from build123d import *

# Parameters (mm, degrees)
SKETCH1_W               = 82.55
SKETCH1_H               = 31.75
BOSS_EXTRUDE1_DEPTH     = 45.72
SHELL1_T                = -1.524
SKETCH3_W               = 25.4
SKETCH3_H               = 5.842
BOSS_EXTRUDE3_DEPTH     = 1.524
FILLET2_R               = 1.27
FILLET3_R               = 1.905
F_2_CLEARANCE_HOLE1_D   = 2.4384
SKETCH6_W               = 44.196
SKETCH6_H               = 28.702
CUT_EXTRUDE1_DEPTH      = 82.026
CUT_EXTRUDE1_DEPTH_BACK = 2.524
FILLET4_R               = 3.556
FILLET5_R               = 5.08
BOSS_EXTRUDE4_DEPTH     = 1.524
FILLET9_R               = 2.54
FILLET10_R              = 2.54


with BuildPart() as part:
    # Sketch1 → Boss-Extrude1 (new body)
    with BuildSketch(Plane.XY):
        Rectangle(SKETCH1_W, SKETCH1_H)
    extrude(amount=BOSS_EXTRUDE1_DEPTH)

    # Shell1
    shell1_openings = [part.faces().sort_by_distance(p)[0] for p in [
        (0, 0, 0),
    ]]
    offset(amount=SHELL1_T, openings=shell1_openings, kind=Kind.INTERSECTION)

    # Sketch3 → Boss-Extrude3 (add)
    with BuildSketch(Plane(origin=(0, 0, 0), x_dir=(-1, 0, 0), z_dir=(0, 0, -1))):
        with Locations((0, 18.796)):
            Rectangle(SKETCH3_W, SKETCH3_H)
        with Locations((0, -18.796)):
            Rectangle(SKETCH3_W, SKETCH3_H)
    extrude(amount=-BOSS_EXTRUDE3_DEPTH)

    # Fillet2
    fillet2_edges = [part.edges().sort_by_distance(p)[0] for p in [
        (12.7, 15.875, 0.762),
        (0, 15.875, 1.524),
        (-12.7, 15.875, 0.762),
        (0, -15.875, 1.524),
        (12.7, -15.875, 0.762),
        (-12.7, -15.875, 0.762),
    ]]
    fillet(fillet2_edges, radius=FILLET2_R)

    # Fillet3
    fillet3_edges = [part.edges().sort_by_distance(p)[0] for p in [
        (12.7, 21.717, 0.762),
        (-12.7, 21.717, 0.762),
        (12.7, -21.717, 0.762),
        (-12.7, -21.717, 0.762),
    ]]
    fillet(fillet3_edges, radius=FILLET3_R)

    # #2 Clearance Hole1 (through all)
    with Locations(Plane.XY.offset(1.524)):
        with Locations((0, 19.431), (0, -19.431)):
            Hole(F_2_CLEARANCE_HOLE1_D / 2)

    # Sketch6 → Cut-Extrude1 (cut, two sides)
    with BuildSketch(Plane(origin=(-39.751, 0, 0), x_dir=(0, 0, -1), z_dir=(1, 0, 0))) as cut_extrude1_sk:
        with Locations((-22.098, 0)):
            Rectangle(SKETCH6_W, SKETCH6_H)
    extrude(amount=CUT_EXTRUDE1_DEPTH, mode=Mode.SUBTRACT)
    extrude(cut_extrude1_sk.sketch, amount=-CUT_EXTRUDE1_DEPTH_BACK, mode=Mode.SUBTRACT)

    # Fillet4
    fillet4_edges = [part.edges().sort_by_distance(p)[0] for p in [
        (0, -14.351, 44.196),
        (0, 14.351, 44.196),
    ]]
    fillet(fillet4_edges, radius=FILLET4_R)

    # Fillet5
    fillet5_edges = [part.edges().sort_by_distance(p)[0] for p in [
        (0, 15.875, 45.72),
        (0, -15.875, 45.72),
    ]]
    fillet(fillet5_edges, radius=FILLET5_R)

    # Sketch7 → Boss-Extrude4 (add)
    with BuildSketch(Plane(origin=(41.275, 0, 0), x_dir=(0, 0, -1), z_dir=(1, 0, 0))):
        with BuildLine():
            Line((-45.72, 10.795), (-45.72, -10.795))
            ThreePointArc((-45.72, -10.795), (-44.232102448, -14.387102448), (-40.64, -15.875))
            Line((-40.64, -15.875), (0, -15.875))
            Line((0, -15.875), (0, -8.89))
            Line((0, -8.89), (-44.196, -8.89))
            Line((-44.196, -8.89), (-44.196, 8.89))
            Line((-44.196, 8.89), (0, 8.89))
            Line((0, 8.89), (0, 15.875))
            Line((0, 15.875), (-40.64, 15.875))
            ThreePointArc((-40.64, 15.875), (-44.232102448, 14.387102448), (-45.72, 10.795))
        make_face()
    boss_extrude4 = extrude(amount=-BOSS_EXTRUDE4_DEPTH)

    # Fillet9
    fillet9_edges = [part.edges().sort_by_distance(p)[0] for p in [
        (40.513, 8.89, 44.196),
        (40.513, -8.89, 44.196),
    ]]
    fillet(fillet9_edges, radius=FILLET9_R)

    # Mirror1: Boss-Extrude4 across plane
    add(boss_extrude4.mirror(Plane(origin=(0, 0, 0), x_dir=(0, 0, 1), z_dir=(1, 0, 0))))

    # Fillet10
    fillet10_edges = [part.edges().sort_by_distance(p)[0] for p in [
        (-40.513, -8.89, 44.196),
        (-40.513, 8.89, 44.196),
    ]]
    fillet(fillet10_edges, radius=FILLET10_R)


solid = part.part
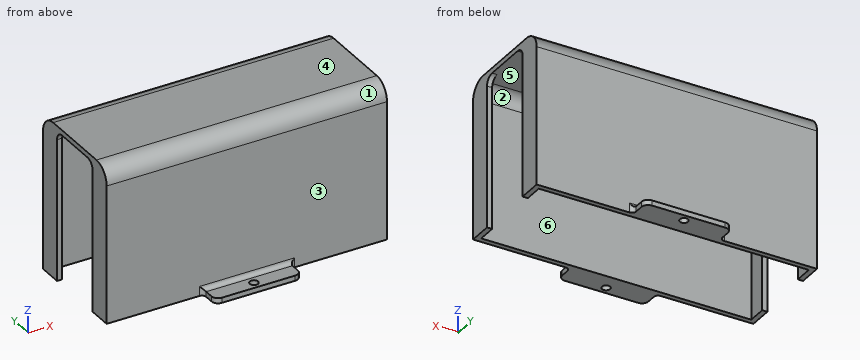
Geometry: final body of the model. Coordinates: model frame, mm. Face numbers are marked on the shaded views. A direction names the side the tool comes from. Coordinates: 2 decimals unless noted, no trailing zeros. Write each loop counter-clockwise with the first axis right and the second up, starting at its lowest first coordinate (ties: lowest second). Pieces come first, ordered by that corner, then holes. Notation, with made-up numbers: (55, 55) - (105, 55) arc R23 ccw to (105, 67) - close; hole circle Ø5 at (51, 52.25). An arc over 180 degrees is marked (long way). Return JSON: item names as keys, results as strings.
Item 1: Pin query (flat end, axial travel): pin 1 Ø3 at (x, y) = (0, -19.431) entering from +Z; pin 2 Ø2 at (y, z) = (7, 38) entering from +X; pin 3 Ø4 at (x, z) = (-24.5, 16.5) entering from -Y (3 decimals); pin 4 Ø0.8 at (y, z) = (19, 0.5) entering from +X. Return the tip coordinate at first contact, or that it passes through.
Completed:
{"pin 1": "stops at z = 1.52", "pin 2": "passes through", "pin 3": "stops at y = -15.875", "pin 4": "stops at x = 12.7"}
Item 2: Section query C-C (x = 31.5). Output: boundary loops of the cut face in (y, z) (3 decimals), and give its area (3 significant figures).
Completed:
{"outline": "(-15.875, 0) - (-14.351, 0) - (-14.351, 40.64) arc R3.556 cw to (-10.795, 44.196) - (10.795, 44.196) arc R3.556 cw to (14.351, 40.64) - (14.351, 0) - (15.875, 0) - (15.875, 40.64) arc R5.08 ccw to (10.795, 45.72) - (-10.795, 45.72) arc R5.08 ccw to (-15.875, 40.64) - close", "area": "177 mm2"}
Item 3: Reachability of the marked faces 1 and 2 from +Z, -Z, +X, -X, +Y, -Y: full face, straight path, thin tool, end or side. Return the list, or none.
Completed:
{"face 1": "+Z, +X, -X, -Y", "face 2": "-Z"}
Item 4: Section query A-A (x = 0). Output: boundary loops of the cut face in (y, z) (3 decimals).
Completed:
{"outline": "(-21.717, 0) - (-20.65, 0) - (-20.65, 1.524) - (-21.717, 1.524) - close; (-18.212, 0) - (-14.351, 0) - (-14.351, 40.64) arc R3.556 cw to (-10.795, 44.196) - (10.795, 44.196) arc R3.556 cw to (14.351, 40.64) - (14.351, 0) - (18.212, 0) - (18.212, 1.524) - (17.145, 1.524) arc R1.27 cw to (15.875, 2.794) - (15.875, 40.64) arc R5.08 ccw to (10.795, 45.72) - (-10.795, 45.72) arc R5.08 ccw to (-15.875, 40.64) - (-15.875, 2.794) arc R1.27 cw to (-17.145, 1.524) - (-18.212, 1.524) - close; (20.65, 0) - (21.717, 0) - (21.717, 1.524) - (20.65, 1.524) - close"}
Item 5: Pull-direction query (Y, two-part tool) for the marked faces 3, 4, 5 and 6; classes: +Y half, -Y half, draft (parallel to the pull), parting line (faces both ways), or undercut.
Completed:
{"face 3": "-Y half", "face 4": "draft", "face 5": "undercut", "face 6": "undercut"}
Item 6: Section query B-B (z = 12). Output: boundary loops of the cut face in (x, y) (3 decimals), and give its area (3 significant figures).
Completed:
{"outline": "(-41.275, -15.875) - (41.275, -15.875) - (41.275, -8.89) - (39.751, -8.89) - (39.751, -14.351) - (-39.751, -14.351) - (-39.751, -8.89) - (-41.275, -8.89) - close; (-41.275, 8.89) - (-39.751, 8.89) - (-39.751, 14.351) - (39.751, 14.351) - (39.751, 8.89) - (41.275, 8.89) - (41.275, 15.875) - (-41.275, 15.875) - close", "area": "285 mm2"}
Item 7: Line query: L1, parallel to Y at x = 0, z = 1; L2, parallel to Y at x = 10.5, z = 22.5 (3 decimals); L3, parallel to X at y = -11.5, z = 19 (3 decimals). Output: solid intervals per line, ascending.
Completed:
{"L1": "y = -21.72 to -20.65, -18.21 to -14.35, 14.35 to 18.21, 20.65 to 21.72", "L2": "y = -15.875 to -14.351, 14.351 to 15.875", "L3": "x = -41.275 to -39.751, 39.751 to 41.275"}
Item 8: Section query D-D (y = 8). Output: boundary loops of the cut face in (x, z) (3 decimals), and give its area (3 significant figures).
Completed:
{"outline": "(-41.275, 43.587) - (-39.751, 43.587) - (-39.751, 44.196) - (39.751, 44.196) - (39.751, 43.587) - (41.275, 43.587) - (41.275, 45.72) - (-41.275, 45.72) - close", "area": "128 mm2"}
